The drawing under review shows one solid part. Ordinate dimensions are in mm from its lowest x, y, z. A direction names the side the tool comes from. Give positions to 0.01 mm unless a question says otherwise; leave off trailing zeros. Write each loop counter-clockwise with the first axis right and the second up, starting at its lowest first coordinate (ties: lowest second). Pieces come first, ordered by that corner, then holes. Notation, with made-up numbers: (44.5, 84.25) -> (62.5, 84.25) arc R7 cw to (62.5, 95.25) -> close; hole circle Ø6 at (28, 20). An arc over 180 degrees is marked (long way). Use CSV: the item, a comma, the result in double quotes.
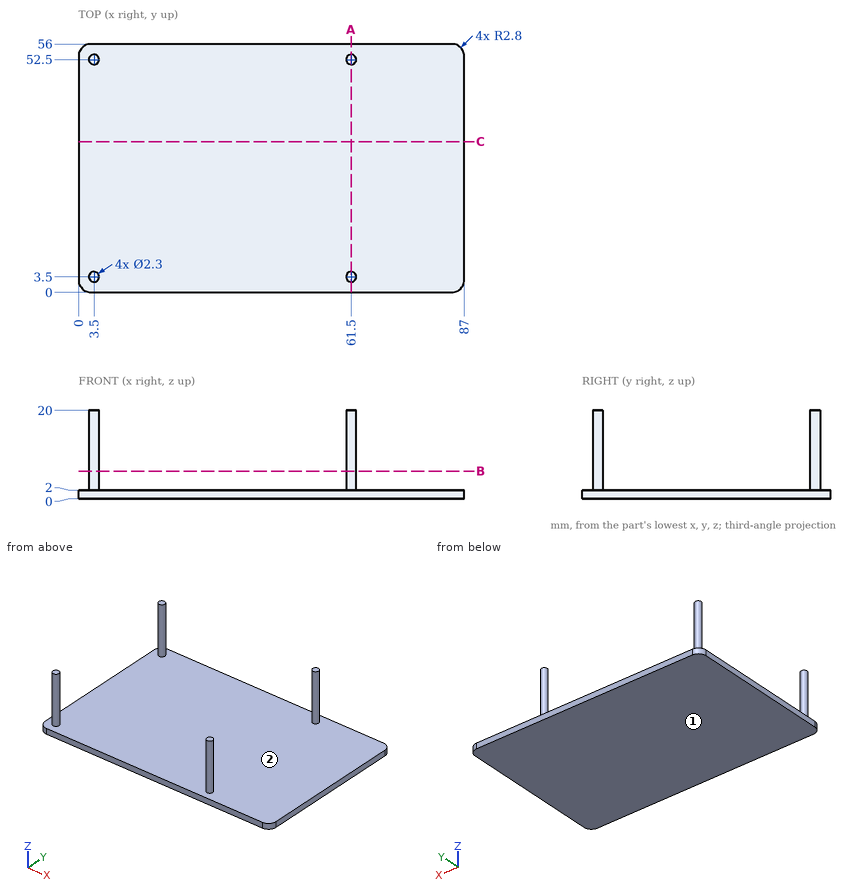
(1) For line 1 along Y through (x, z) = (61.5, 6.5); line 2 along Z through (x, y) = (9, 53.5); line 3 along X through (y, z) = (53, 15.25), list the stretches that pass through material, from the lowest coordinate up. Write a range as [from, to].
Established:
line 1,"y = [2.35, 4.65], [51.35, 53.65]"
line 2,"z = [0, 2]"
line 3,"x = [2.46, 4.54], [60.46, 62.54]"
(2) Clearance check with flat-ended pins moving along their axes: pin 1 (10 mm diameter, centred on y = 20, z = 11, fed in from +X); pin 2 (12 mm diameter, centred on x = 40, y = 35, fed in from +Z). State where each tip first meets the part, or that it passes through.
Established:
pin 1,"passes through"
pin 2,"stops at z = 2"
(3) Take a section at A-A (x = 61.5). Write out the cut boundary in (y, z).
Established:
outline,"(0, 0) -> (56, 0) -> (56, 2) -> (53.65, 2) -> (53.65, 20) -> (51.35, 20) -> (51.35, 2) -> (4.65, 2) -> (4.65, 20) -> (2.35, 20) -> (2.35, 2) -> (0, 2) -> close"
(4) Tool access review of the marked faces 1 and 2: name each direction out of +Z, -Z, +X, -X, +Y, -Y from which nothing blocks a thin tool from reaching the whole face with its end or side.
Established:
face 1,"-Z, +X, -X, +Y, -Y"
face 2,"+Z"
(5) Take a section at B-B (z = 6.25). Write out the cut boundary in (x, y).
Established:
outline,"circle Ø2.3 at (3.5, 3.5); circle Ø2.3 at (3.5, 52.5); circle Ø2.3 at (61.5, 3.5); circle Ø2.3 at (61.5, 52.5)"
(6) Take a section at C-C (y = 34). Write out the cut boundary in (x, z), then the cut area to 3 significant figures.
Established:
outline,"(0, 0) -> (87, 0) -> (87, 2) -> (0, 2) -> close"
area,"174 mm2"
